Can you work these out from the model? Positions are in its coordinate system, mm. Face numbers are marked on the shaded views. A direction names the side the tool comes from. Coordinates: 2 decimals unless noted, no trailing zeros. Order: outer loops, then holes, each group sorted by start corner. A loop starts at its lowest first (then second) coordinate and runs counter-clockwise, first axis right, second up. Notation, with made-up numbers: (63, 30.5) -> (72, 30.5) arc R21 ccw to (72, 50.5) -> close; hole circle Ø9 at (-3.75, -33). An arc over 180 degrees is marked (long way). Return JSON: item names as keys, results as strings. Group by question number.
1) If we section it at A-A, the plane z = 13: Please give me the cut outline in (x, y).
2) For pin 1 (6 mm diameter, centred on x = 25, y = -111, fed in from +Z); pin 2 (5 mm diameter, centred on y = -108.5, z = 11.5, fed in from +X); pin 3 (1 mm diameter, centred on y = -114.5, z = 13, fed in from -X), each with a flat end and sliding along its axis, tell me the tip position at first contact or that it passes through.
3) For the marked faces 4, 5 and 6, which set-ups out of +Z, -Z, +X, -X, +Y, -Y let a thin tool reach every point of the face, with its end or its side?
4) If I drill on probe 1 along X at (y, z) = (-111, 1.2); probe 2 along Y at (x, z) = (25, 3.5); probe 3 along X at (y, z) = (-114.5, 13.5), over which ranges is the centre line in solid material (lowest first)? Write a range as from..to.
5) Thinking about a two-plate mould opening in X: for the marked faces 1, 2 and 3, which applies, +X half, -X half, draft (parallel to the pull), parting line (faces both ways), or undercut?
6) If we section it at C-C, the plane y = -111: State how many separate pieces and enclosed holes the cut face has, then the cut area to 3 significant figures.
7) If we section it at B-B, the plane x = 15: Please give me the cut outline in (y, z).
from build123d import *

# Parameters (mm, degrees)
SKETCH_1_W          = 111
SKETCH_1_H          = 10
SKETCH_1_R          = 1.8
EXTRUDE_1_DEPTH     = 4.75
SKETCH_2_W          = 4
SKETCH_2_H          = 10
EXTRUDE_2_DEPTH     = 15.5
SKETCH_3_W          = 4.5
SKETCH_3_H          = 10
EXTRUDE_3_DEPTH     = 14
SKETCH_4_W          = 4.5
SKETCH_4_H          = 10
EXTRUDE_4_DEPTH     = 14
FILLET_1_R          = 5
FILLET_2_R          = 1
SKETCH_5_W          = 20
SKETCH_5_H          = 2
CUT_EXTRUDE_1_DEPTH = 14
FILLET_4_R          = 3
FILLET_5_R          = 2
CUT_EXTRUDE_2_DEPTH = 200
FILLET_6_R          = 0.5
FILLET_7_R          = 1


with BuildPart() as part:
    # ｽｹｯﾁ1 → ﾎﾞｽ - 押し出し1 (new body)
    with BuildSketch(Plane.XY):
        with Locations((0, -111)):
            Rectangle(SKETCH_1_W, SKETCH_1_H)
        with Locations((25, -111)):
            Circle(SKETCH_1_R, mode=Mode.SUBTRACT)
        with Locations((15, -111)):
            Circle(SKETCH_1_R, mode=Mode.SUBTRACT)
        with Locations((-15, -111)):
            Circle(SKETCH_1_R, mode=Mode.SUBTRACT)
        with Locations((-25, -111)):
            Circle(SKETCH_1_R, mode=Mode.SUBTRACT)
    extrude(amount=EXTRUDE_1_DEPTH)

    # ｽｹｯﾁ2 → ﾎﾞｽ - 押し出し2 (add)
    with BuildSketch(Plane.XY.offset(4.75)):
        with Locations((39.5, -111)):
            Rectangle(SKETCH_2_W, SKETCH_2_H)
        with Locations((-39.5, -111)):
            Rectangle(SKETCH_2_W, SKETCH_2_H)
    extrude(amount=EXTRUDE_2_DEPTH)

    # ｽｹｯﾁ3 → ﾎﾞｽ - 押し出し3 (add)
    with BuildSketch(Plane(origin=(41.5, 0, 0), x_dir=(0, 0, -1), z_dir=(1, 0, 0))):
        with Locations((-18, -111)):
            Rectangle(SKETCH_3_W, SKETCH_3_H)
    extrude(amount=EXTRUDE_3_DEPTH)

    # ｽｹｯﾁ4 → ﾎﾞｽ - 押し出し4 (add)
    with BuildSketch(Plane.ZY.offset(41.5)):
        with Locations((18, -111)):
            Rectangle(SKETCH_4_W, SKETCH_4_H)
    extrude(amount=EXTRUDE_4_DEPTH)

    # ﾌｨﾚｯﾄ1
    fillet_1_edges = [part.edges().sort_by_distance(p)[0] for p in [
        (37.5, -111, 4.75),
        (-37.5, -111, 4.75),
    ]]
    fillet(fillet_1_edges, radius=FILLET_1_R)

    # ﾌｨﾚｯﾄ2
    fillet_2_edges = [part.edges().sort_by_distance(p)[0] for p in [
        (37.5, -111, 20.25),
        (-37.5, -111, 20.25),
        (-55.5, -111, 0),
        (55.5, -111, 20.25),
        (55.5, -111, 0),
        (-55.5, -111, 20.25),
    ]]
    fillet(fillet_2_edges, radius=FILLET_2_R)

    # ｽｹｯﾁ5 → ｶｯﾄ - 押し出し1 (cut)
    with BuildSketch(Plane(origin=(0, -106, 0), x_dir=(1, 0, 0), z_dir=(0, 1, 0))):
        with Locations((0, -3.75)):
            Rectangle(SKETCH_5_W, SKETCH_5_H)
    extrude(amount=-CUT_EXTRUDE_1_DEPTH, mode=Mode.SUBTRACT)

    # ﾌｨﾚｯﾄ4
    # the kernel refuses this fillet: 3 mm, written as the material it adds along each edge
    with BuildSketch(Plane(origin=(10, -106, 2.75), x_dir=(-1, 0, 0), z_dir=(0, -1, 0))) as fillet_4_piece_1:
        with BuildLine():
            CenterArc((2.828427125, -3), FILLET_4_R, 90, 70.528779366)
            Line((0, -2), (-0.056568542, -1.98))
            ThreePointArc((-0.056568542, -1.98), (-0.06, -1), (-0.06, 0))
            Line((-0.06, 0), (0, 0.06))
            Line((0, 0.06), (2.828427125, 0.06))
            Line((2.828427125, 0.06), (2.828427125, 0))
        make_face()
    extrude(amount=10)
    with BuildSketch(Plane(origin=(-10, -106, 2.75), x_dir=(0, 0, 1), z_dir=(0, -1, 0))) as fillet_4_piece_2:
        with BuildLine():
            CenterArc((3, -2.828427125), FILLET_4_R, 109.471220634, 70.528779366)
            Line((0, -2.828427125), (-0.06, -2.828427125))
            Line((-0.06, -2.828427125), (-0.06, 0))
            Line((-0.06, 0), (0, 0.06))
            ThreePointArc((0, 0.06), (1, 0.06), (1.98, 0.056568542))
            Line((1.98, 0.056568542), (2, 0))
        make_face()
    extrude(amount=10)

    # ﾌｨﾚｯﾄ5
    fillet_5_edges = [part.edges().sort_by_distance(p)[0] for p in [
        (-10, -111, 4.75),
        (10, -111, 4.75),
    ]]
    fillet(fillet_5_edges, radius=FILLET_5_R)

    # ｽｹｯﾁ6 → ｶｯﾄ - 押し出し2 (cut)
    with BuildSketch(Plane(origin=(0, -106, 0), x_dir=(1, 0, 0), z_dir=(0, 1, 0))):
        Polygon((-55.5, -4.75), (-48.5, -4.75), (-55.5, -3.25), align=None)
        Polygon((-41.5, -4.75), (-41.5, -3.25), (-48.5, -4.75), align=None)
        Polygon((-41.5, -15.75), (-48.5, -15.75), (-41.5, -17.25), align=None)
        Polygon((-55.5, -17.25), (-48.5, -15.75), (-55.5, -15.75), align=None)
        Polygon((55.5, -4.75), (55.5, -3.25), (48.5, -4.75), align=None)
        Polygon((41.5, -4.75), (48.5, -4.75), (41.5, -3.25), align=None)
        Polygon((55.5, -15.75), (48.5, -15.75), (55.5, -17.25), align=None)
        Polygon((41.5, -15.75), (41.5, -17.25), (48.5, -15.75), align=None)
    extrude(amount=-CUT_EXTRUDE_2_DEPTH, mode=Mode.SUBTRACT)

    # ﾌｨﾚｯﾄ6
    fillet_6_edges = [part.edges().sort_by_distance(p)[0] for p in [
        (-55.5, -111, 17.25),
        (48.5, -111, 15.75),
        (-48.5, -111, 4.75),
        (-55.5, -111, 3.25),
        (-48.5, -111, 15.75),
        (48.5, -111, 4.75),
        (55.5, -111, 3.25),
        (55.5, -111, 17.25),
    ]]
    fillet(fillet_6_edges, radius=FILLET_6_R)

    # ﾌｨﾚｯﾄ7
    fillet_7_edges = [part.edges().sort_by_distance(p)[0] for p in [
        (41.5, -111, 17.25),
        (-41.5, -111, 3.25),
        (-41.5, -111, 17.25),
        (41.5, -111, 3.25),
    ]]
    fillet(fillet_7_edges, radius=FILLET_7_R)


solid = part.part
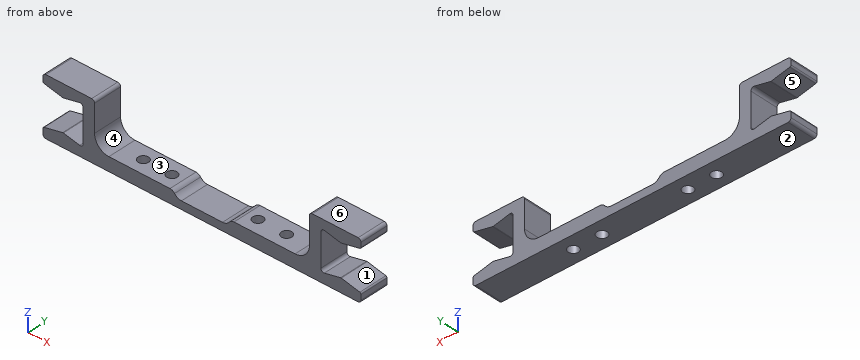
Result sheet:
{
 "1": {"outline": "(-41.5, -116) -> (-37.5, -116) -> (-37.5, -106) -> (-41.5, -106) -> close; (37.5, -116) -> (41.5, -116) -> (41.5, -106) -> (37.5, -106) -> close"},
 "2": {"pin 1": "stops at z = 4.75", "pin 2": "stops at x = 41.5", "pin 3": "stops at x = -41.5"},
 "3": {"face 4": "+Z, +Y, -Y", "face 5": "-X, +Y, -Y", "face 6": "+Z, +X, -X, +Y, -Y"},
 "4": {"probe 1": "x = -55.5..-26.8, -23.2..-16.8, -13.2..13.2, 16.8..23.2, 26.8..55.5", "probe 2": "y = -116..-112.8, -109.2..-106", "probe 3": "x = -41.5..-37.5, 37.5..41.5"},
 "5": {"face 1": "+X half", "face 2": "draft", "face 3": "undercut"},
 "6": {"separate pieces": "5", "enclosed holes": "0", "area": "640 mm2"},
 "7": {"outline": "(-116, 0) -> (-112.8, 0) -> (-112.8, 4.75) -> (-116, 4.75) -> close; (-109.2, 0) -> (-106, 0) -> (-106, 4.75) -> (-109.2, 4.75) -> close"}
}
